Check sheet for the modelled part. Datum: model origin and axes. Units: mm. Coordinates: 2 decimals unless noted, no trailing zeros. Write each loop counter-clockwise with the first axis right and the second up, starting at its lowest first coordinate (ties: lowest second). Pieces come first, ordered by that corner, then holes. Notation, with made-up numbers: (-34.5, -34) - (-5.5, -34) arc R22 cw to (-5.5, -14) - close; hole circle Ø9 at (57.25, 64.5). An arc over 180 degrees is marked (long way). Use one line per item in the form item = value. Start each with the question number.
1. Scan lines: line 1 along Y through (x, z) = (-27.5, 0.5); line 2 along X through (y, z) = (-0.5, 0.85); line 3 along X through (y, z) = (0.75, 0.6). Record each from-to range of solid material in increasing order.
2. Cross-section at C-C on y = -3.25. Record the boundary of the cut face in (x, z), then the cut area to 3 significant figures.
3. Cross-section at B-B on x = 0. Record the boundary of the cut face in (y, z).
4. Cross-section at A-A on z = 1. Give the number of separate pieces and of enclosed holes in the cut face, then the cut area to 3 significant figures.
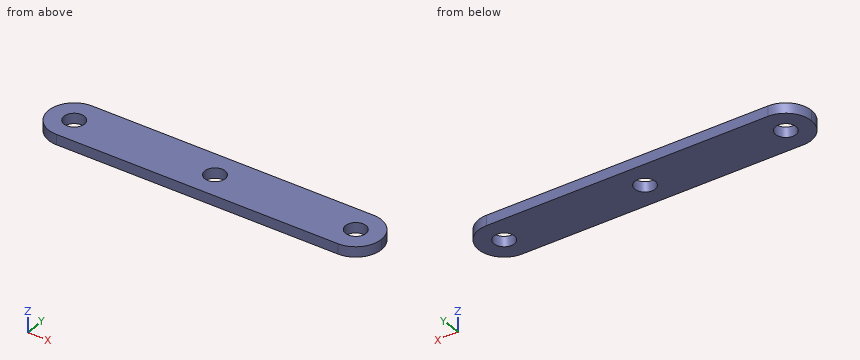
```python
from build123d import *

# Parameters (mm, degrees)
SKETCH_1_W          = 65
SKETCH_1_H          = 10
EXTRUDE_1_DEPTH     = 2
FILLET_1_R          = 5
SKETCH_3_R          = 2
CUT_EXTRUDE_1_DEPTH = 2


with BuildPart() as part:
    # 草图1 → 凸台-拉伸1 (new body)
    with BuildSketch(Plane.XY):
        Rectangle(SKETCH_1_W, SKETCH_1_H)
    extrude(amount=EXTRUDE_1_DEPTH)

    # 圆角1
    fillet_1_edges = [part.edges().sort_by_distance(p)[0] for p in [
        (32.5, -5, 1),
        (-32.5, -5, 1),
        (-32.5, 5, 1),
        (32.5, 5, 1),
    ]]
    fillet(fillet_1_edges, radius=FILLET_1_R - 0.0001)  # a hair under: the kernel refuses the full size

    # 草图3 → 切除-拉伸1 (cut)
    with BuildSketch(Plane.XY.offset(2)):
        with Locations((-27.5, 0)):
            Circle(SKETCH_3_R)
        with Locations(Location((27.5, 0, 0), (0, 0, 180))):
            Circle(SKETCH_3_R)
        Circle(SKETCH_3_R)
    extrude(amount=-CUT_EXTRUDE_1_DEPTH, mode=Mode.SUBTRACT)


solid = part.part
```
Final values:
q1.line_1 = -5 to -2, 2 to 5
q1.line_2 = -32.47 to -29.44, -25.56 to -1.94, 1.94 to 25.56, 29.44 to 32.47
q1.line_3 = -32.44 to -29.35, -25.65 to -1.85, 1.85 to 25.65, 29.35 to 32.44
q2.outline = (-31.3, 0) - (31.3, 0) - (31.3, 2) - (-31.3, 2) - close
q2.area = 125 mm²
q3.outline = (-5, 0) - (-2, 0) - (-2, 2) - (-5, 2) - close; (2, 0) - (5, 0) - (5, 2) - (2, 2) - close
q4.separate_pieces = 1
q4.enclosed_holes = 3
q4.area = 591 mm²
